from build123d import *

# Parameters (mm, degrees)
F0_W     = 12.319
F0_H     = 19.939
F1_DEPTH = 50.8
F2_T     = -1.27
F3_R     = 1.26999
F4_W     = 6.604
F4_H     = 6.604
F5_DEPTH = 5.842


# Not quite as in the source:
# - a fillet or chamfer is up to 0.001 mm smaller than in the source, because OpenCascade refuses the exact size


with BuildPart() as f1:
    # F0 (on Top) → F1 (new body)
    with BuildSketch(Plane.XY):
        Rectangle(F0_W, F0_H)
    extrude(amount=F1_DEPTH)

    # F2
    f2_openings = [f1.faces().sort_by_distance(p)[0] for p in [
        (0, 0, 50.8),
    ]]
    offset(amount=F2_T, openings=f2_openings)

    # F3 (radius 1.27 in the source; OpenCascade refuses exactly that, so slightly less here)
    f3_edges = [f1.edges().sort_by_distance(p)[0] for p in [
        (0, -9.9695, 50.8),
        (6.1595, 0, 50.8),
        (0, 9.9695, 50.8),
        (-6.1595, 0, 50.8),
        (-6.1595, -9.9695, 25.4),
        (6.1595, -9.9695, 25.4),
        (6.1595, 9.9695, 25.4),
        (-6.1595, 9.9695, 25.4),
    ]]
    fillet(f3_edges, radius=F3_R)

    # F4 (on face) → F5 (join)
    with BuildSketch(Plane(origin=(0, 0, 0), x_dir=(1, 0, 0), z_dir=(0, 0, -1))):
        Rectangle(F4_W, F4_H)
    extrude(amount=F5_DEPTH)


solid = f1.part
Can you work these out from the model? Positions are in its coordinate system, mm. A direction names the side the tool comes from. Coordinates: 2 decimals unless noted, no trailing zeros. Write each loop counter-clockwise with the first axis right and the second up, starting at its lowest first coordinate (ties: lowest second). Pieces come first, ordered by that corner, then holes. Notation, with made-up numbers: (70, 12.5) -> (127, 12.5) arc R19 ccw to (127, 44.5) -> close; hole circle Ø11 at (56, -5.75). An arc over 180 degrees is marked (long way). Write each question's results on one line, items separated by ' | '. Start each with the question number.
Item 1: Thinking about a two-plate mould opening in Y: for faces 1 (the flat face through (0, -3.302, -3)), 2 (the flat face through (0, 0, 1.27)), 3 (the flat face through (3.302, 0, -3)), which applies, released by +Y, released by -Y, zero draft, split by the parting line, or undercut?
Item 2: Please list where these lines run through material, in increasing order: probe 1 along X at (y, z) = (6.75, 13.5); probe 2 along Y at (x, z) = (1.5, 7.5); probe 3 along Z at (x, y) = (-4, -1.25).
Item 3: On a 3-axis mill with a long thin cutter (end or side, diameter ignored), from which of +Z, -Z, +X, -X, +Y, -Y can I reach the whole of each face in a straight line? I mean faces 4 (the flat face through (0, 3.302, -3)), 5 (the flat face through (-3.302, 0, -3)), 6 (the cylindrical face through (0.068, -9.607, 50.418)), 7 (the flat face through (4.89, 0, 26)). Say none if no direction works.
Item 4: If we section it at A-A, the plane z = 38.5: Write out the boundary of the cut face in (x, y).
Item 5: I'm going to push flat-ended pins straight in: P1, Ø5, axis at x = 0, y = 3.5, coming from the +Z side; P2, Ø3, axis at x = -0.5, z = -4, coming from the -Y side; P3, Ø4.5, axis at x = 1.5, z = -3.5, coming from the +Y side. Where does each tip first touch, or does it pass through?
Answer block:
1) face 1: released by -Y | face 2: undercut | face 3: zero draft
2) probe 1: -6.16 to -4.89, 4.89 to 6.16 | probe 2: -9.97 to -8.7, 8.7 to 9.97 | probe 3: 0 to 1.27
3) face 4: -Z, +X, -X, +Y | face 5: -Z, -X, +Y, -Y | face 6: +Z, +X, -X, -Y | face 7: +Z
4) outline: (-6.16, -8.7) arc R1.27 ccw to (-4.89, -9.97) -> (4.89, -9.97) arc R1.27 ccw to (6.16, -8.7) -> (6.16, 8.7) arc R1.27 ccw to (4.89, 9.97) -> (-4.89, 9.97) arc R1.27 ccw to (-6.16, 8.7) -> close; hole (-4.89, -8.7) -> (4.89, -8.7) -> (4.89, 8.7) -> (-4.89, 8.7) -> close
5) P1: z = 1.27 | P2: y = -3.3 | P3: y = 3.3
